Could you check a few things on this drawing? It's one solid part, dimensions in mm from its lowest x, y, z. Give positions to 0.01 mm unless a question says otherwise; leave off trailing zeros. Order: outer loops, then holes, each group sorted by start corner. A loop starts at its lowest first (then second) coordinate and runs counter-clockwise, first axis right, second up. Notation, with made-up numbers: (33, -5.75) - (49, -5.75) arc R20 ccw to (49, 27.25) - close; hole circle Ø2 at (-30, -23.75). An arc over 180 degrees is marked (long way). Put each result on its own line as item: value.
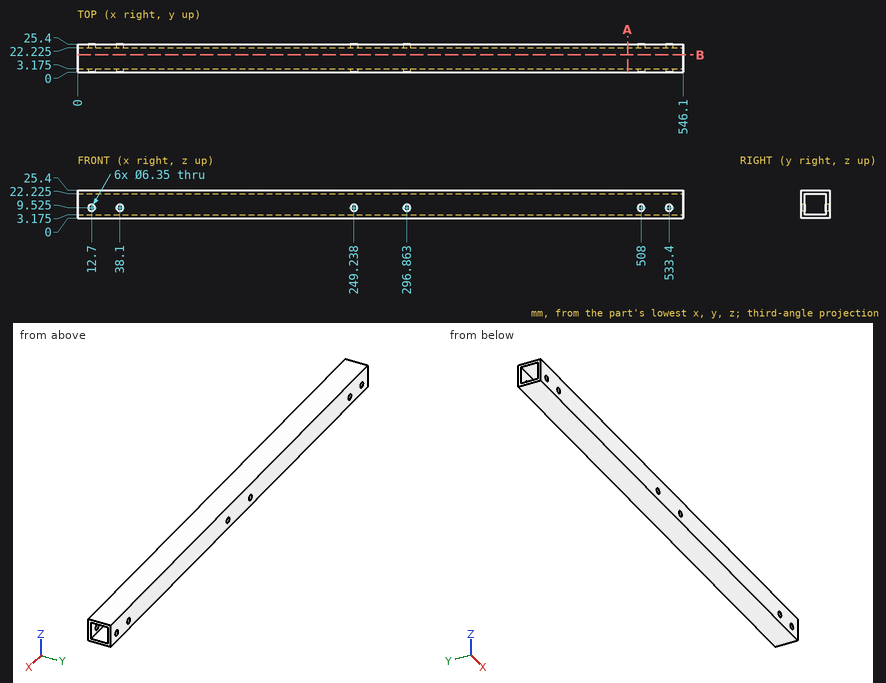
1) I'm going to push a flat-ended pin straight in: pin 1 (6 mm diameter, centred on y = 10.5, z = 5.5, fed in from -X). Where does the tip first touch, or does it pass through?
Filled in:
pin 1: stops at x = 0
2) If I drill on line 1 (Z direction, x = 12.7, y = 2); line 2 (Z direction, x = 447, y = 11) (1 decimal), over which ranges is the centre line in solid material (lowest first)? Write a range as [from, to].
Filled in:
line 1: z = [0, 6.35], [12.7, 25.4]
line 2: z = [0, 3.2], [22.2, 25.4]
3) Suppose I cut it at B-B, the plane y = 15.5. List the corners of the cut face in (x, z) for me (1 decimal), and give its area (3 significant figures).
Filled in:
outline: (0, 0) - (546.1, 0) - (546.1, 3.2) - (0, 3.2) - close; (0, 22.2) - (546.1, 22.2) - (546.1, 25.4) - (0, 25.4) - close
area: 3,470 mm^2
4) Suppose I cut it at A-A, the plane x = 496. List the corners of the cut face in (y, z) for me (1 decimal), and give its area (3 significant figures).
Filled in:
outline: (0, 0) - (25.4, 0) - (25.4, 25.4) - (0, 25.4) - close; hole (3.2, 3.2) - (22.2, 3.2) - (22.2, 22.2) - (3.2, 22.2) - close
area: 282 mm^2
